Part model, mm, in its own coordinate system. A direction names the side the tool comes from. Coordinates: 2 decimals unless noted, no trailing zeros. Loops run counter-clockwise (first coordinate to the right, second up) from the corner with the lowest first, then second, coordinate; pieces in that order, holes last. Notation, with made-up numbers: (51.5, 75) -> (80.5, 75) arc R21 cw to (80.5, 96) -> close; hole circle Ø1 at (-13.5, -13). An arc over 180 degrees is marked (long way). Use one line per item in the form item = value. Start each with the question number.
(1) Pin check, flat tips, straight feed: P1, Ø4, axis at y = 276.5, z = -6.5, coming from the +X side; P2, Ø8, axis at x = -12.5, z = -10, coming from the -Y side. Stop position of each tip, or through.
(2) Mould opens along X. For faces 1 (the flat face through (-13, 455, -15.871)), 2 (the flat face through (-13, 455, -17.395)), 3 (the flat face through (-25.4, 458, -5)) say: +X half, -X half, draft (parallel to the pull), parting line (faces both ways), or undercut.
(3) Band-saw the part on B-B on y = 522.5. Give the cut face in (x, z).
(4) 3-axis set-ups, long thin cutter, end or side, ignore diameter. For faces 4 (the flat face through (-12.759, 873.675, 6.653)), 5 (the flat face through (-13, 455, 6.481)): which of +Z, -Z, +X, -X, +Y, -Y reach the whole face in a straight line?
(5) Drill centre lines: L1, parallel to X at y = 221.5, z = -12.25; L2, parallel to Z at x = -22.25, y = 163. Where is each one in solid material? Low to high. Write a range as [from, to].
(6) Band-saw the part on C-C on x = -18.5. Give the cut face in (y, z).
(7) Band-saw the part on A-A on z = -2.25. Give the cut face in (x, y).
```python
from build123d import *

# Parameters (mm, degrees)
SKETCH1_W               = 25.4
SKETCH1_H               = 25.4
SKETCH1_W_2             = 22.352
SKETCH1_H_2             = 22.352
BOSS_EXTRUDE1_DEPTH     = 877.062
CUT_EXTRUDE1_DEPTH      = 1
CUT_EXTRUDE1_DEPTH_BACK = 26.4
CUT_EXTRUDE2_DEPTH      = 1
CUT_EXTRUDE2_DEPTH_BACK = 26.4


with BuildPart() as part:
    # Sketch1 → Boss-Extrude1 (new body)
    with BuildSketch(Plane(origin=(0, 0, 0), x_dir=(1, 0, 0), z_dir=(0, 1, 0))):
        with Locations((-12.7, 4.695189487)):
            Rectangle(SKETCH1_W, SKETCH1_H)
        with Locations((-12.7, 4.695189487)):
            Rectangle(SKETCH1_W_2, SKETCH1_H_2, mode=Mode.SUBTRACT)
    extrude(amount=BOSS_EXTRUDE1_DEPTH)

    # Sketch2 → Cut-Extrude1 (cut, two sides)
    with BuildSketch(Plane.XY.offset(8.004810513)) as cut_extrude1_sk:
        Polygon((-25.4, 877.062), (0, 870.256090512), (0, 877.062), align=None)
    extrude(amount=CUT_EXTRUDE1_DEPTH, mode=Mode.SUBTRACT)
    extrude(cut_extrude1_sk.sketch, amount=-CUT_EXTRUDE1_DEPTH_BACK, mode=Mode.SUBTRACT)

    # Sketch3 → Cut-Extrude2 (cut, two sides)
    with BuildSketch(Plane(origin=(0, 0, -17.395189487), x_dir=(-1, 0, 0), z_dir=(0, 0, -1))) as cut_extrude2_sk:
        Polygon((25.4, 0), (25.4, 50.8), (0, 43.994090512), (0, 0), align=None)
    extrude(amount=CUT_EXTRUDE2_DEPTH, mode=Mode.SUBTRACT)
    extrude(cut_extrude2_sk.sketch, amount=-CUT_EXTRUDE2_DEPTH_BACK, mode=Mode.SUBTRACT)


solid = part.part
```
A:
q1.P1 = 0
q1.P2 = through
q2.face_1 = undercut
q2.face_2 = draft
q2.face_3 = -X half
q3.outline = (-25.4, -17.4) -> (0, -17.4) -> (0, 8) -> (-25.4, 8) -> close; hole (-23.88, -15.87) -> (-1.52, -15.87) -> (-1.52, 6.48) -> (-23.88, 6.48) -> close
q4.face_4 = +Z, -Z, +X, +Y
q4.face_5 = +Y, -Y
q5.L1 = [-25.4, -23.88], [-1.52, 0]
q5.L2 = [-17.4, -15.87], [6.48, 8]
q6.outline = (48.95, -17.4) -> (875.21, -17.4) -> (875.21, -15.87) -> (48.95, -15.87) -> close; (48.95, 6.48) -> (875.21, 6.48) -> (875.21, 8) -> (48.95, 8) -> close
q7.outline = (-25.4, 50.8) -> (-23.88, 50.39) -> (-23.88, 876.65) -> (-25.4, 877.06) -> close; (-1.52, 44.4) -> (0, 43.99) -> (0, 870.26) -> (-1.52, 870.66) -> close
